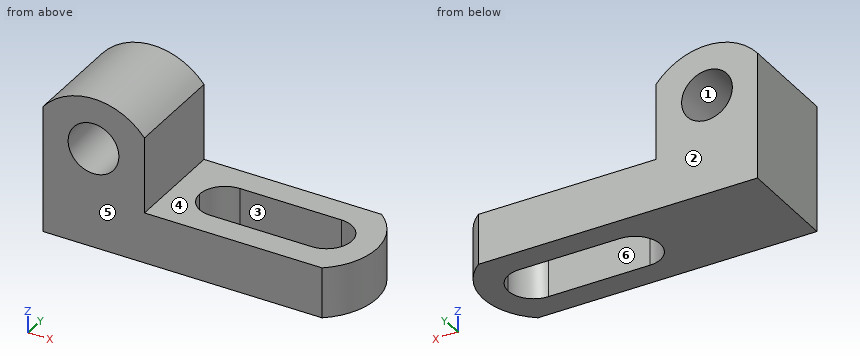
```python
from build123d import *

# Parameters (mm, degrees)
F1_DEPTH = 25.4
F3_DEPTH = 25.4
F5_DEPTH = 25.4
F6_R     = 6.35
F7_DEPTH = 25.4
F9_DEPTH = 25.4


with BuildPart() as f1:
    # F0 (on Front) → F1 (new body)
    with BuildSketch(Plane.XZ):
        Polygon((0, 38.1), (0, 0), (76.2, 0), (76.2, 12.7), (25.4, 12.7), (25.4, 38.1), align=None)
    extrude(amount=F1_DEPTH)

    # F2 (on face) → F3 (cut)
    with BuildSketch(Plane.XZ.offset(25.4)):
        with BuildLine():
            Line((0, 38.1), (0, 31.75))
            ThreePointArc((0, 31.75), (12.7, 37.721269), (25.4, 31.75))
            Line((25.4, 31.75), (25.4, 38.1))
            Line((25.4, 38.1), (0, 38.1))
        make_face()
    extrude(amount=-F3_DEPTH, mode=Mode.SUBTRACT)

    # F4 (on face) → F5 (cut)
    with BuildSketch(Plane.XY.offset(12.7)):
        with BuildLine():
            Line((63.5, -6.35), (38.1, -6.35))
            ThreePointArc((38.1, -6.35), (33.609872, -8.209872), (31.75, -12.7))
            ThreePointArc((31.75, -12.7), (33.609872, -17.190128), (38.1, -19.05))
            Line((38.1, -19.05), (63.5, -19.05))
            ThreePointArc((63.5, -19.05), (67.990128, -17.190128), (69.85, -12.7))
            ThreePointArc((69.85, -12.7), (67.990128, -8.209872), (63.5, -6.35))
        make_face()
    extrude(amount=-F5_DEPTH, mode=Mode.SUBTRACT)

    # F6 (on face) → F7 (cut)
    with BuildSketch(Plane.XZ.offset(25.4)):
        with Locations((12.644723, 25.02139)):
            Circle(F6_R)
    extrude(amount=-F7_DEPTH, mode=Mode.SUBTRACT)

    # F8 (on face) → F9 (cut)
    with BuildSketch(Plane.XY.offset(12.7)):
        with BuildLine():
            Line((76.2, 0), (69.85, 0))
            ThreePointArc((69.85, 0), (76.095109, -12.7), (69.85, -25.4))
            Line((69.85, -25.4), (76.2, -25.4))
            Line((76.2, -25.4), (76.2, 0))
        make_face()
    extrude(amount=-F9_DEPTH, mode=Mode.SUBTRACT)


solid = f1.part
```
Check sheet for the modelled part. Datum: model origin and axes. Units: mm. Face numbers are marked on the shaded views. A direction names the side the tool comes from. Give positions to 0.01 mm unless a question says otherwise; leave off trailing zeros. Write each loop counter-clockwise with the first axis right and the second up, starting at its lowest first coordinate (ties: lowest second). Pieces come first, ordered by that corner, then holes. Notation, with made-up numbers: (-13, 43.25) - (24, 43.25) arc R26 ccw to (24, 62.25) - close; hole circle Ø6 at (19.5, 34). An arc over 180 degrees is marked (long way). Answer as a JSON object with one key per item and string values. Group by question number.
1) Sectioned sample at A-A (y = -8.5). Record the cut outline in (x, z).
2) Depth check by flat-ended pin: P1, Ø2, axis at y = -9, z = 16, coming from the +X side; P2, Ø3, axis at x = 49, y = -20, coming from the +Z side. Enter the tip coordinate at first touch or a pass-through.
3) Sectioned sample at C-C (x = 39). Record the cut outline in (y, z), then the cut area to 3 significant figures.
4) Thickness scan on probe 1 along Y at (x, z) = (45.5, 7.5); probe 2 along X at (y, z) = (-15.25, 15); probe 3 along Y at (x, z) = (37.5, 11). Record the ranges inside material, lowest first. Write a range as from..to.
5) Sectioned sample at D-D (z = 21). Record the cut outline in (x, y), then the cut area to 3 significant figures.
6) Sectioned sample at B-B (z = 10.5). Record the cut outline in (x, y), then the cut area to 3 significant figures.
7) Release check for a two-part mould opening along Y. For the marked faces 1, 2 and 3 record: pulls with the +Y half, pulls with the -Y half, needs draft (parallel to the pull), parting line crosses it, or undercut.
8) Access from +Z, -Z, +X, -X, +Y, -Y to the whole of each face (thin tool, end or side, straight path). Record for the marked faces 4, 5 and 6.
Geometry results:
{
 "1": {"outline": "(0, 0) - (33.34, 0) - (33.34, 12.7) - (25.4, 12.7) - (25.4, 31.75) arc R16.49 ccw to (0, 31.75) - close; (68.26, 0) - (75.54, 0) - (75.54, 12.7) - (68.26, 12.7) - close; hole circle Ø12.7 at (12.64, 25.02)"},
 "2": {"P1": "stops at x = 25.4", "P2": "stops at z = 12.7"},
 "3": {"outline": "(-25.4, 0) - (-19.05, 0) - (-19.05, 12.7) - (-25.4, 12.7) - close; (-6.35, 0) - (0, 0) - (0, 12.7) - (-6.35, 12.7) - close", "area": "161 mm^2"},
 "4": {"probe 1": "y = -25.4..-19.05, -6.35..0", "probe 2": "x = 0..25.4", "probe 3": "y = -25.4..-19.02, -6.38..0"},
 "5": {"outline": "(0, -25.4) - (7.73, -25.4) - (7.73, 0) - (0, 0) - close; (17.56, -25.4) - (25.4, -25.4) - (25.4, 0) - (17.56, 0) - close", "area": "396 mm^2"},
 "6": {"outline": "(0, -25.4) - (69.85, -25.4) arc R16.04 ccw to (69.85, 0) - (0, 0) - close; hole (38.1, -19.05) - (63.5, -19.05) arc R6.35 ccw to (63.5, -6.35) - (38.1, -6.35) arc R6.35 ccw to start", "area": "1,440 mm^2"},
 "7": {"face 1": "needs draft", "face 2": "pulls with the +Y half", "face 3": "undercut"},
 "8": {"face 4": "+Z, +X, +Y, -Y", "face 5": "+Z, -Z, +X, -X, -Y", "face 6": "+Z, -Z"}
}
